Part model, mm, in its own coordinate system. Face numbers are marked on the shaded views. A direction names the side the tool comes from. Round coordinates to 2 decimals unless told otherwise and drop trailing zeros. Loops run counter-clockwise (first coordinate to the right, second up) from the corner with the lowest first, then second, coordinate; pieces in that order, holes last. Notation, with made-up numbers: (10.5, 45.5) - (21.5, 45.5) arc R23 ccw to (21.5, 58.5) - close; hole circle Ø2 at (-32, 11.25). An arc over 180 degrees is marked (long way). Write each question's results on one line, items separated by ' | '. Start each with the question number.
(1) Drill centre lines: L1, parallel to X at y = 100, z = 113; L2, parallel to Y at x = 9, z = 53.5; L3, parallel to Z at x = -36, y = 104.5. Where is each one in solid material? Low to high.
(2) Mould opens along Z. For the marked faces 1, 2, 3 and 4 say: released by +Z, released by -Z, zero draft, split by the parting line, or undercut.
(3) Cut at C-C, the plane y = 100. List the corners of the cut face in (x, z).
(4) Flat gauge pin, fed straight in: P1, Ø3, axis at x = -0.5, z = -24, coming from the -Y side. Where does the tip first touch, or does it go through?
(5) Tool access for the marked faces 5 and 6: list every direction of +Z, -Z, +X, -X, +Y, -Y with a clear straight run to the whole face (end or side of a thin tool).
(6) Cut at A-A, the plane x = -37. List the corners of the cut face in (y, z).
(7) Cut at B-B, the plane z = 111.5. List the corners of the cut face in (x, y), then the cut area to 3 significant figures.
(8) Cut at D-D, the plane z = 61. List the corners of the cut face in (x, y).
from build123d import *

# Parameters (mm, degrees)
SKETCH1_W           = 200
SKETCH1_H           = 200
BOSS_EXTRUDE1_DEPTH = 200
SKETCH2_R           = 50
CUT_EXTRUDE2_DEPTH  = 210
SKETCH4_R           = 50
CUT_EXTRUDE3_DEPTH  = 100


with BuildPart() as part:
    # Sketch1 → Boss-Extrude1 (new body)
    with BuildSketch(Plane(origin=(0, 0, 0), x_dir=(1, 0, 0), z_dir=(0, 1, 0))):
        with Locations((38.271604938, -41.975308642)):
            Rectangle(SKETCH1_W, SKETCH1_H)
    extrude(amount=BOSS_EXTRUDE1_DEPTH)

    # Sketch2 → Cut-Extrude2 (cut)
    with BuildSketch(Plane.ZY.offset(61.728395062)):
        with Locations((41.975308642, 100)):
            Circle(SKETCH2_R)
    extrude(amount=-CUT_EXTRUDE2_DEPTH, mode=Mode.SUBTRACT)

    # Sketch4 → Cut-Extrude3 (cut)
    with BuildSketch(Plane.XY.offset(141.975308642)):
        with Locations((38.271604938, 100)):
            Circle(SKETCH4_R)
    extrude(amount=-CUT_EXTRUDE3_DEPTH, mode=Mode.SUBTRACT)


solid = part.part
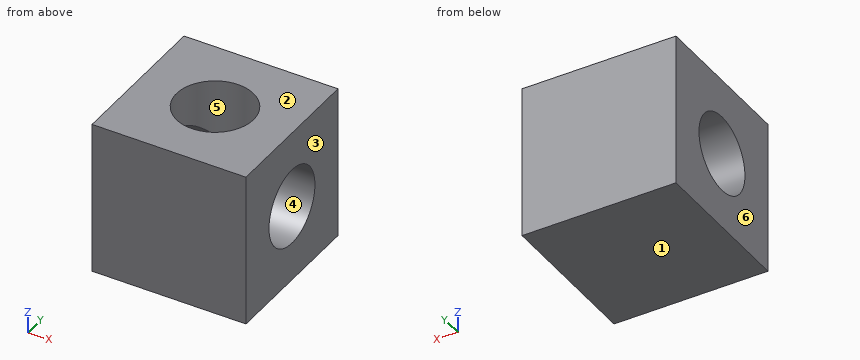
A:
1) L1: -61.73 to -11.73, 88.27 to 138.27 | L2: 0 to 51.35, 148.65 to 200 | L3: -58.02 to -7.82, 91.77 to 141.98
2) face 1: released by -Z | face 2: released by +Z | face 3: zero draft | face 4: undercut
3) outline: (-61.73, -58.02) - (138.27, -58.02) - (138.27, -8.02) - (-61.73, -8.02) - close; (-61.73, 91.98) - (-11.73, 91.98) - (-11.73, 141.98) - (-61.73, 141.98) - close; (88.27, 91.98) - (138.27, 91.98) - (138.27, 141.98) - (88.27, 141.98) - close
4) P1: y = 0
5) face 5: +Z | face 6: +Z, -Z, -X, +Y, -Y
6) outline: (0, -58.02) - (200, -58.02) - (200, 141.98) - (0, 141.98) - close; hole circle Ø100 at (100, 41.98)
7) outline: (-61.73, 0) - (138.27, 0) - (138.27, 200) - (-61.73, 200) - close; hole circle Ø100 at (38.27, 100) | area: 32,100 mm2
8) outline: (-61.73, 0) - (138.27, 0) - (138.27, 53.76) - (57.3, 53.76) arc R50 cw to (19.25, 53.76) - (-61.73, 53.76) - close; (-61.73, 146.24) - (19.25, 146.24) arc R50 cw to (57.3, 146.24) - (138.27, 146.24) - (138.27, 200) - (-61.73, 200) - close
